Check sheet for the modelled part. Datum: model origin and axes. Units: mm. A direction names the side the tool comes from. Round coordinates to 2 decimals unless told otherwise and drop trailing zeros. Order: outer loops, then holes, each group sorted by start corner. A loop starts at its lowest first (then second) coordinate and runs counter-clockwise, first axis right, second up. Notation, with made-up numbers: (38, 25.25) -> (63, 25.25) arc R27 ccw to (63, 43.25) -> close; hole circle Ø11 at (39, 87.25). An arc over 180 degrees is marked (long way). Answer as CSV lines item,"result". Start each with the question number.
from build123d import *

# Parameters (mm, degrees)
SKETCH1_W           = 40
SKETCH1_H           = 20
BOSS_EXTRUDE1_DEPTH = 40
SKETCH2_W           = 20
SKETCH2_H           = 20
BOSS_EXTRUDE2_DEPTH = 40
CUT_EXTRUDE1_DEPTH  = 20


with BuildPart() as part:
    # Sketch1 → Boss-Extrude1 (new body)
    with BuildSketch(Plane.XY):
        with Locations((20, 10)):
            Rectangle(SKETCH1_W, SKETCH1_H)
    extrude(amount=BOSS_EXTRUDE1_DEPTH)

    # Sketch2 → Boss-Extrude2 (add)
    with BuildSketch(Plane.XY.offset(40)):
        with Locations((30, 30)):
            Rectangle(SKETCH2_W, SKETCH2_H)
    extrude(amount=-BOSS_EXTRUDE2_DEPTH)

    # Sketch3 → Cut-Extrude1 (cut)
    with BuildSketch(Plane(origin=(0, 40, 0), x_dir=(1, 0, 0), z_dir=(0, 1, 0))):
        Polygon((20, 0), (20, -20), (40, 0), align=None)
        Polygon((40, -40), (20, -20), (20, -40), align=None)
    extrude(amount=-CUT_EXTRUDE1_DEPTH, mode=Mode.SUBTRACT)


solid = part.part
1) Section check C-C on y = 30. Record the cut outline in (x, z).
2) Material ranges on line 1 along Y through (x, z) = (6, 7.5); line 2 along X through (y, z) = (34, 7.5); line 3 along X through (y, z) = (32, 6.5), recorded low to high.
3) Section check A-A on x = 33. Record the cut outline in (y, z).
4) Access from +Z, -Z, +X, -X, +Y, -Y to the whole of each face (thin tool, end or side, straight path). Record for faces 1 (the face through (30, 30, 30)), 2 (the face through (0, 10, 20)), 3 (the face through (30, 30, 10)).
5) Depth check by flat-ended pin: pin 1 Ø3 at (x, y) = (27, 26.5) entering from +Z; pin 2 Ø8 at (y, z) = (29.5, 6.5) entering from -X; pin 3 Ø1 at (x, z) = (23, 11.5) entering from +Y; pin 4 Ø12 at (x, z) = (19, 30.5) entering from -Y. Enter the tip coordinate at first touch or a pass-through.
6) Section check B-B on z = 37. Record the cut outline in (x, y), then the cut area to 3 significant figures.
7) Section check D-D on z = 10. Record the cut outline in (x, y).
Solutions:
1,outline,"(20, 20) -> (40, 0) -> (40, 40) -> close"
2,line 1,"y = 0 to 20"
2,line 2,"x = 32.5 to 40"
2,line 3,"x = 33.5 to 40"
3,outline,"(0, 0) -> (20, 0) -> (20, 7) -> (40, 7) -> (40, 33) -> (20, 33) -> (20, 40) -> (0, 40) -> close"
4,face 1,"+Z, -X, +Y"
4,face 2,"+Z, -Z, -X, +Y, -Y"
4,face 3,"-Z, -X, +Y"
5,pin 1,"stops at z = 28.5"
5,pin 2,"stops at x = 29.5"
5,pin 3,"stops at y = 20"
5,pin 4,"stops at y = 0"
6,outline,"(0, 0) -> (40, 0) -> (40, 40) -> (37, 40) -> (37, 20) -> (0, 20) -> close"
6,area,"860 mm^2"
7,outline,"(0, 0) -> (40, 0) -> (40, 40) -> (30, 40) -> (30, 20) -> (0, 20) -> close"
